Geometry: see drawing. Coordinates: mm, zero at the bounding-box minimum. Round coordinates to 2 decimals unless told otherwise and drop trailing zeros. Order: outer loops, then holes, each group sorted by start corner. A loop starts at its lowest first (then second) coordinate and runs counter-clockwise, first axis right, second up. Notation, with made-up numbers: (-8, 32) -> (35, 32) arc R14 ccw to (35, 49) -> close; hole circle Ø7 at (49, 55). An arc over 180 degrees is marked (long way). Write item = value, one per line. Start each with the question number.
(1) Cut plane A-A on x = 63. Return the cut outline in (y, z).
(2) Cut plane C-C on y = 43.5. Return the cut outline in (x, z).
(3) Ray query, line 1 (X direction, y = 39, z = 1.15); line 2 (X direction, y = 23, z = 1.55); line 3 (X direction, y = 56.5, z = 0.4) (1 decimal). Return the intervals inside material, ascending.
(4) Cut plane B-B on z = 0.45. Return the cut outline in (x, y), then the cut area to 3 significant figures.
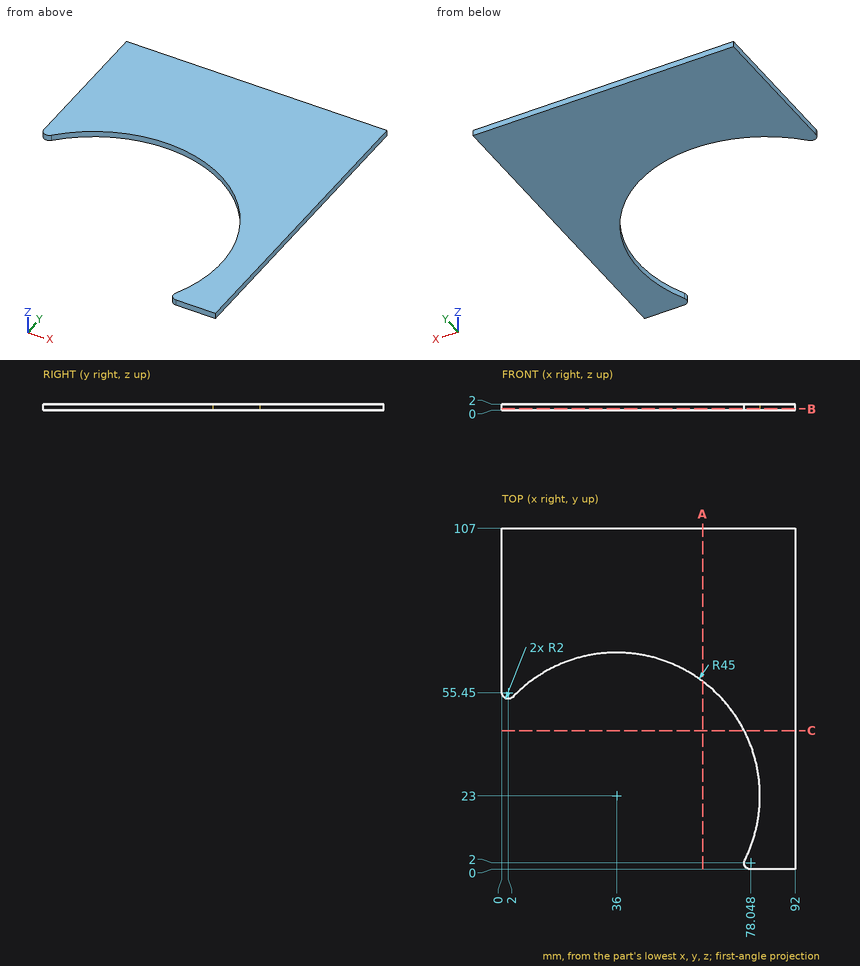
Evaluation:
q1.outline = (59, 0) -> (107, 0) -> (107, 2) -> (59, 2) -> close
q2.outline = (76.06, 0) -> (92, 0) -> (92, 2) -> (76.06, 2) -> close
q3.line_1 = 78.06 to 92
q3.line_2 = 81 to 92
q3.line_3 = 0 to 6, 66 to 92
q4.outline = (0, 55.45) arc R2 ccw to (3.45, 54.07) arc R45 cw to (76.26, 2.89) arc R2 ccw to (78.05, 0) -> (92, 0) -> (92, 107) -> (0, 107) -> close
q4.area = 5,000 mm^2
